Autodesk Inventor part; units mm, degrees
ref_plane "YZ Plane" through (0, 0, 0) normal (1, 0, 0) x (0, 1, 0)
ref_plane "XZ Plane" through (0, 0, 0) normal (0, 1, 0) x (-1, 0, 0)
ref_plane "XY Plane" through (0, 0, 0) normal (0, 0, 1) x (1, 0, 0)
sketch "Sketch1" plane through (0, 0, 0) normal (0, 1, 0) x (-1, 0, 0)
  line L0 (-2.15, -3.2) -> (2.15, -3.2)
  line L1 (2.15, -3.2) -> (2.15, 3.2)
  line L2 (2.15, 3.2) -> (-2.15, 3.2)
  line L3 (-2.15, 3.2) -> (-2.15, -3.2)
  line L4 (-2.15, -3.2) -> (2.15, 3.2) construction
  line L5 (2.15, -3.2) -> (-2.15, 3.2) construction
  point P0 (0, 0)
  dimension "d0" = 6.4
  dimension "d1" = 4.3
extrude "Extrusion1" add sketch "Sketch1" along normal blind 2.6
sketch "Sketch2" plane through (0, 2.6, 0) normal (0, 1, 0) x (1, 0, 0)
  line L0 (2.15, -3.2) -> (2.15, 3.2)
  line L1 (2.15, -1.2) -> (0.55, -1.2)
  line L2 (2.15, 1.2) -> (0.55, 1.2)
  arc A0 (0.55, 1.2) -> (0.55, -1.2) centre (0.55, 0) ccw
  point P0 (0, 0)
  dimension "d4" = 2.4
  dimension "d5" = 1.2
  dimension "d6" = 1.6
  dimension "d7" = 1.2
extrude "Extrusion2" cut sketch "Sketch2" against normal through all
fillet "Fillet1" radius 0.1 6 edges at (2.15, 1.3, 3.2) (-2.15, 1.3, 3.2) (-2.15, 1.3, -3.2) (2.15, 1.3, -3.2) (2.15, 1.3, -1.2) (2.15, 1.3, 1.2)
properties part number "Edge Spacer v2p0"
Build history of the part. All positions in model axes, mm. Round coordinates to 2 decimals unless told otherwise and drop trailing zeros. Order: outer loops, then holes, each group sorted by start corner. A loop starts at its lowest first (then second) coordinate and runs counter-clockwise, first axis right, second up. Notation, with made-up numbers: (17.5, -37) -> (43.5, -37) arc R25 ccw to (43.5, -1) -> close; hole circle Ø6 at (4, 21). An arc over 180 degrees is marked (long way). Answer in a Markdown table with one row per item.
1) Pin check, flat tip, straight feed: P1, Ø2, axis at x = 1, z = -1, coming from the -Y side. Stop position of the tip, or through.
Values:
| item | result |
|---|---|
| P1 | y = 0 |
2) Wall check: L1, parallel to Z at x = 1.5, y = 1.65; L2, parallel to Z at x = -0.5, y = 2.1; L3, parallel to X at y = 1, z = 0. Give the ranges that are in metal, low to high.
Values:
| item | result |
|---|---|
| L1 | -3.2 to -1.2, 1.2 to 3.2 |
| L2 | -3.2 to -0.58, 0.58 to 3.2 |
| L3 | -2.15 to -0.65 |
3) Band-saw the part on A-A on x = 1.2. Give the cut face in (y, z).
Values:
| item | result |
|---|---|
| outline | (0, -3.2) -> (2.6, -3.2) -> (2.6, -1.2) -> (0, -1.2) -> close; (0, 1.2) -> (2.6, 1.2) -> (2.6, 3.2) -> (0, 3.2) -> close |
4) Mould opens along Z. For faces 1 (the flat face through (1, 1, -1.2)), 2 (the flat face through (0, 1, 3.2)), 3 (the flat face through (2.15, 1, 2)), 4 (the flat face through (1, 1, 1.2)) say: released by +Z, released by -Z, zero draft, split by the parting line, or undercut.
Values:
| item | result |
|---|---|
| face 1 | undercut |
| face 2 | released by +Z |
| face 3 | zero draft |
| face 4 | undercut |
5) Band-saw the part on C-C on z = 0. Give the cut face in (x, y), and give its area (3 significant figures).
Values:
| item | result |
|---|---|
| outline | (-2.15, 0) -> (-0.65, 0) -> (-0.65, 2.6) -> (-2.15, 2.6) -> close |
| area | 3.90 mm2 |
6) Band-saw the part on D-D on z = 1. Give the cut face in (x, y).
Values:
| item | result |
|---|---|
| outline | (-2.15, 0) -> (-0.11, 0) -> (-0.11, 2.6) -> (-2.15, 2.6) -> close |
7) Band-saw the part on B-B on y = 2.35. Give the cut face in (x, z), and give its area (3 significant figures).
Values:
| item | result |
|---|---|
| outline | (-2.15, -3.1) arc R0.1 ccw to (-2.05, -3.2) -> (2.05, -3.2) arc R0.1 ccw to (2.15, -3.1) -> (2.15, -1.3) arc R0.1 ccw to (2.05, -1.2) -> (0.55, -1.2) arc R1.2 cw to (0.55, 1.2) -> (2.05, 1.2) arc R0.1 ccw to (2.15, 1.3) -> (2.15, 3.1) arc R0.1 ccw to (2.05, 3.2) -> (-2.05, 3.2) arc R0.1 ccw to (-2.15, 3.1) -> close |
| area | 21.4 mm2 |
